from build123d import *

# Parameters (mm, degrees)
SKETCH_3_R          = 6.5
SKETCH_3_R_2        = 5.1
EXTRUDE_1_DEPTH     = 7
SKETCH_4_R          = 8
CUT_EXTRUDE_1_DEPTH = 5


with BuildPart() as part:
    # 草图3 → 凸台-拉伸1 (new body)
    with BuildSketch(Plane.XY):
        with BuildLine():
            Line((-22.387222404, 6.481913971), (-37.741822074, 15.137156625))
            ThreePointArc((-37.741822074, 15.137156625), (-44.677179157, 17.972501845), (-52.098826017, 19.000858921))
            ThreePointArc((-52.098826017, 19.000858921), (-62.839328708, 31.635038635), (-48.859263412, 40.553484096))
            ThreePointArc((-48.859263412, 40.553484096), (-42.068238936, 39.382208167), (-35.189110999, 39.791475278))
            Line((-35.189110999, 39.791475278), (6.380330607, 47.121287778))
            ThreePointArc((6.380330607, 47.121287778), (12.780626397, 49.003020007), (18.606824384, 52.252653742))
            ThreePointArc((18.606824384, 52.252653742), (34.217539735, 49.304351078), (30.601923927, 33.834566184))
            ThreePointArc((30.601923927, 33.834566184), (24.699361424, 29.262109391), (20.108758873, 23.373648349))
            Line((20.108758873, 23.373648349), (16.20338738, 16.820058769))
            ThreePointArc((16.20338738, 16.820058769), (12.916733667, 8.922247815), (11.992720655, 0.417913012))
            ThreePointArc((11.992720655, 0.417913012), (3.095129334, -11.593971468), (-10.60533968, -5.614870459))
            ThreePointArc((-10.60533968, -5.614870459), (-15.627603439, 1.279586072), (-22.387222404, 6.481913971))
        make_face()
        with Locations((-51.961523087, 30.000001974)):
            Circle(SKETCH_3_R, mode=Mode.SUBTRACT)
        with Locations((25.000001645, 43.30126924)):
            Circle(SKETCH_3_R, mode=Mode.SUBTRACT)
        Circle(SKETCH_3_R_2, mode=Mode.SUBTRACT)
        with BuildLine():
            Line((6.06060926, 43.804004569), (-34.143508536, 37.139474198))
            ThreePointArc((-34.143508536, 37.139474198), (-38.136023536, 33.571352415), (-36.611887481, 28.438256042))
            ThreePointArc((-36.611887481, 28.438256042), (-34.460833245, 26.729480075), (-32.162485272, 25.224639143))
            Line((-32.162485272, 25.224639143), (-30.686333973, 24.351977435))
            ThreePointArc((-30.686333973, 24.351977435), (-7.018632683, 21.377002096), (11.337823614, 36.610224829))
            ThreePointArc((11.337823614, 36.610224829), (10.909838082, 41.82878296), (6.06060926, 43.804004569))
        make_face(mode=Mode.SUBTRACT)
    extrude(amount=EXTRUDE_1_DEPTH)

    # 草图4 → 切除-拉伸1 (cut)
    with BuildSketch(Plane(origin=(0, 0, 0), x_dir=(-1, 0, 0), z_dir=(0, 0, -1))):
        Circle(SKETCH_4_R)
    extrude(amount=-CUT_EXTRUDE_1_DEPTH, mode=Mode.SUBTRACT)


solid = part.part
Can you work these out from the model? Positions are in its coordinate system, mm. A direction names the side the tool comes from. Give positions to 0.01 mm unless a question says otherwise; leave off trailing zeros. Loops run counter-clockwise (first coordinate to the right, second up) from the corner with the lowest first, then second, coordinate; pieces in that order, holes last. Notation, with made-up numbers: M 49,17.25 L 99,17.25 A27 cw 99,47.25 Z; hole C -14,34 d1. An arc over 180 degrees is marked long. One line per item, written item: value. Start each with the question number.
1) I'm going to push flat-ended pins straight in: pin 1 (2 mm diameter, centred on x = -10.5, z = 1.5, fed in from -Y); pin 2 (5 mm diameter, centred on x = 3, y = -1, fed in from -Z); pin 3 (1.5 mm diameter, centred on x = -35.5, z = 5.5, fed in from -Y). Where does each tip first touch, or does it pass through?
2) If we section it at A-A, the plane x = -17.5: Write out the boundary of the cut face in (y, z).
3) If we section it at B-B, the plane z = 3.5: Write out the boundary of the cut face in (x, y), and give its area (3 significant figures).
4) Thinking about a two-plate mould opening in Y: for faces 1 (the face through (-62.875, 31.375, 3.451)), 2 (the face through (-13.76, 40.52, 3.45)), 3 (the face through (-15.54, 1.19, 3.45)), which applies, +Y half, -Y half, draft (parallel to the pull), parting line (faces both ways), or undercut?
5) On a 3-axis mill with a long thin cutter (end or side, diameter ignored), from which of +Z, -Z, +X, -X, +Y, -Y can I reach the whole of each face in a straight line? I mean faces 4 (the face through (24.774, 29.336, 3.451)), 5 (the face through (-10, 16, 0)), 6 (the face through (-7.349, 21.283, 3.451)), 7 (the face through (-5, -2, 5)), 8 (the face through (-14.695, 43.405, 3.451)). Say none if no direction works.
6) If I drill on line 1 (X direction, y = 33.5, z = 1.25); line 2 (Y direction, x = -52, z = 2); line 3 (X direction, y = 28.5, z = 3.75), over which ranges is the centre line in solid material (lowest first)? Write a range as [from, to].
7) If we section it at C-C, the plane y = 21.5: Write out the boundary of the cut face in (x, z), and give its area (3 significant figures).
8) If we section it at D-D, the plane x = 0: Write out the boundary of the cut face in (y, z), and give its area (3 significant figures).
Completed:
1. pin 1: stops at y = -7.33
1. pin 2: stops at z = 5
1. pin 3: stops at y = 13.45
2. outline: M 3.04,0 L 20.25,0 L 20.25,7 L 3.04,7 Z; M 39.9,0 L 42.91,0 L 42.91,7 L 39.9,7 Z
3. outline: M -52.1,19 A30 cw -37.74,15.14 L -22.39,6.48 A30 cw -10.61,-5.61 A12 ccw 11.99,0.42 A30 cw 16.2,16.82 L 20.11,23.37 A30 cw 30.6,33.83 A11 ccw long 18.61,52.25 A30 cw 6.38,47.12 L -35.19,39.79 A30 cw -48.86,40.55 A11 ccw long Z; hole C -51.96,30 d13; hole M -36.61,28.44 A30 ccw -32.16,25.22 L -30.69,24.35 A30 ccw 11.34,36.61 A5 ccw 6.06,43.8 L -34.14,37.14 A5 ccw Z; hole C 0,0 d16; hole C 25,43.3 d13
3. area: 2,060 mm^2
4. face 1: parting line
4. face 2: undercut
4. face 3: -Y half
5. face 4: +Z, -Z, +X, -Y
5. face 5: -Z, +X, -X, +Y, -Y
5. face 6: +Z, -Z
5. face 7: -Z
5. face 8: +Z, -Z, +Y
6. line 1: x = [-62.39, -57.44], [-46.48, -38.16], [9.52, 30.05]
6. line 2: y = [19, 23.5], [36.5, 41]
6. line 3: x = [-62.86, -58.29], [-45.64, -36.68], [5.32, 23.96]
7. outline: M -58.94,0 L -24.23,0 L -24.23,7 L -58.94,7 Z; M -6.61,0 L 18.99,0 L 18.99,7 L -6.61,7 Z
7. area: 422 mm^2
8. outline: M -12,0 L -8,0 L -8,5 L -5.1,5 L -5.1,7 L -12,7 Z; M 5.1,5 L 8,5 L 8,0 L 24.44,0 L 24.44,7 L 5.1,7 Z; M 42.8,0 L 46,0 L 46,7 L 42.8,7 Z
8. area: 177 mm^2
